from build123d import *

# Parameters (mm, degrees)
F1_DEPTH       = 65.024
F3_D           = 9.525
F3_CBORE_D     = 12.7
F3_CBORE_DEPTH = 6.35
F4_W           = 31.75
F4_H           = 7.112
F5_DEPTH       = 38.1
F6_W           = 7.112
F6_H           = 38.1
F7_DEPTH       = 101.601
F9_DEPTH       = 101.601
F11_D          = 9.525
F11_DEPTH      = 15.875
F11_TIP        = 2.8615986981
F12_W          = 6.604
F12_H          = 6.35
F13_DEPTH      = 101.601
F15_DEPTH      = 101.601
F16_W          = 7.112
F16_H          = 6.35
F17_DEPTH      = 101.601
F18_R          = 9.525
F19_DEPTH      = 31.751


with BuildPart() as f1:
    # F0 (on Front) → F1 (new body)
    with BuildSketch(Plane.XZ):
        Polygon((-50.8, 69.85), (-50.8, 0), (50.8, 0), (50.8, 69.85), (19.05, 69.85), (19.05, 31.75), (-19.05, 31.75), (-19.05, 69.85), align=None)
    extrude(amount=F1_DEPTH)

    # F3 (through all)
    with Locations(Plane.XZ.offset(65.024)):
        with Locations((0, 15.875)):
            CounterBoreHole(F3_D / 2, F3_CBORE_D / 2, F3_CBORE_DEPTH)

    # F4 (on face) → F5 (cut)
    with BuildSketch(Plane.XY.offset(69.85)):
        with Locations((-34.925, -61.468)):
            Rectangle(F4_W, F4_H)
    extrude(amount=-F5_DEPTH, mode=Mode.SUBTRACT)

    # F6 (on face) → F7 (cut, through all)
    with BuildSketch(Plane.YZ.offset(50.8)):
        with Locations((-61.468, 50.8)):
            Rectangle(F6_W, F6_H)
        with Locations((-3.556, 50.8)):
            Rectangle(F6_W, F6_H)
    extrude(amount=-F7_DEPTH, mode=Mode.SUBTRACT)

    # F8 (on face) → F9 (cut, through all)
    with BuildSketch(Plane.YZ.offset(50.8)):
        with BuildLine():
            Line((-12.7, 6.35), (-52.324, 6.35))
            ThreePointArc((-52.324, 6.35), (-56.8141280605, 4.4901280605), (-58.674, 0))
            Line((-58.674, 0), (-6.35, 0))
            ThreePointArc((-6.35, 0), (-8.2098719395, 4.4901280605), (-12.7, 6.35))
        make_face()
    extrude(amount=-F9_DEPTH, mode=Mode.SUBTRACT)

    # F11
    with Locations(Plane.YZ.offset(50.8)):
        with Locations((-32.512, 22.225)):
            Hole(F11_D / 2, depth=F11_DEPTH)
            with Locations((0, 0, -(F11_DEPTH + F11_TIP / 2))):  # 118° drill point
                Cone(0, F11_D / 2, F11_TIP, mode=Mode.SUBTRACT)

    # F12 (on face) → F13 (cut, through all)
    with BuildSketch(Plane.YZ.offset(50.8)):
        with Locations((-32.512, 50.927)):
            Rectangle(F12_W, F12_H)
    extrude(amount=-F13_DEPTH, mode=Mode.SUBTRACT)

    # F14 (on face) → F15 (cut, through all)
    with BuildSketch(Plane.YZ.offset(50.8)):
        Polygon((-50.8, 69.85), (-35.814, 54.102), (-29.21, 54.102), (-14.224, 69.85), align=None)
    extrude(amount=-F15_DEPTH, mode=Mode.SUBTRACT)

    # F16 (on face) → F17 (cut, through all)
    with BuildSketch(Plane.YZ.offset(50.8)):
        with Locations((-10.668, 34.925)):
            Rectangle(F16_W, F16_H)
        with Locations((-54.356, 34.925)):
            Rectangle(F16_W, F16_H)
    extrude(amount=-F17_DEPTH, mode=Mode.SUBTRACT)

    # F18 (on face) → F19 (cut, through all)
    with BuildSketch(Plane.XY.offset(31.75)):
        with Locations((0, -32.512)):
            Circle(F18_R)
    extrude(amount=-F19_DEPTH, mode=Mode.SUBTRACT)


solid = f1.part
The listing builds one solid part. Answer for the finished solid, in the listing's coordinates (mm). A direction names the side the tool comes from. Give positions to 0.01 mm unless a question says otherwise; leave off trailing zeros. Loops run counter-clockwise (first coordinate to the right, second up) from the corner with the lowest first, then second, coordinate; pieces in that order, holes last. Notation, with made-up numbers: M 23,17 L 40,17 A24 ccw 40,56 Z; hole C 86.25,-13 d7. An arc over 180 degrees is marked long. Answer as CSV lines item,"result".
Item 1: Straight lines are drawn through the part: line 1 along Z through (x, y) = (0, -63.5) (3 decimals); line 2 along X through (y, z) = (-22, 16); line 3 along X through (y, z) = (-43.5, 59.5). For each, find the intervals that lie inside material, in ascending order. Write a range as [from, to].
Values follow:
line 1,"z = [0, 9.525], [22.225, 31.75]"
line 2,"x = [-50.8, -4.76], [4.76, 50.8]"
line 3,"x = [-50.8, -19.05], [19.05, 50.8]"
Item 2: The part is cut by section A-A (z = 42.5). Give the vertices of the cut face in (x, y), and give its area (3 significant figures).
Values follow:
outline,"M -50.8,-57.91 L -19.05,-57.91 L -19.05,-7.11 L -50.8,-7.11 Z; M 19.05,-57.91 L 50.8,-57.91 L 50.8,-7.11 L 19.05,-7.11 Z"
area,"3,230 mm^2"
Item 3: The mould has two halves that part along Y. Classify faces 5 (the flat face through (-34.7, -21.82, 61.87)), 6 (the flat face through (35, -7.112, 54)), 7 (the cylindrical face through (4.76, -49.59, 16.08)), 8 (the flat face through (-35, -29.21, 51)): released by +Y, released by -Y, zero draft, split by the parting line, or undercut.
Values follow:
face 5,"undercut"
face 6,"released by +Y"
face 7,"zero draft"
face 8,"undercut"
Item 4: The part is cut by section D-D (z = 58). Give the vertices of the cut face in (x, y).
Values follow:
outline,"M -50.8,-57.91 L -19.05,-57.91 L -19.05,-39.52 L -50.8,-39.52 Z; M -50.8,-25.5 L -19.05,-25.5 L -19.05,-7.11 L -50.8,-7.11 Z; M 19.05,-57.91 L 50.8,-57.91 L 50.8,-39.52 L 19.05,-39.52 Z; M 19.05,-25.5 L 50.8,-25.5 L 50.8,-7.11 L 19.05,-7.11 Z"
Item 5: The part is cut by section C-C (x = 0). Give the number of separate pieces and of enclosed holes in the cut face, and give its area (3 significant figures).
Values follow:
separate pieces,"4"
enclosed holes,"0"
area,"808 mm^2"
Item 6: Which of the six approach directions +Z, -Z, +X, -X, +Y, -Y give full straight-line access (tool end or side, diameter ignored) to faces 1 (the flat face through (-11, -32, 6.35)), 2 (the flat face through (35, -54, 38.1)), 3 (the flat face through (35, -35.814, 51)), 4 (the flat face through (35, -57.912, 54))?
Values follow:
face 1,"-Z, +X, -X"
face 2,"+X, -X, -Y"
face 3,"+Z, +X, -X"
face 4,"+Z, +X, -X, -Y"
Item 7: Given pin 1 Ø10 at (x, z) = (0, 15.875) entering from -Y; pin 2 Ø3 at (x, z) = (-32, 50.5) entering from +Y; pin 3 Ø3.5 at (x, y) = (-42.5, -32) entering from +Z, each flat-ended and moving along its own axis, determine where each tip first touches the part or whether it passes through.
Values follow:
pin 1,"stops at y = -58.67"
pin 2,"stops at y = -7.11"
pin 3,"stops at z = 47.75"
